from build123d import *

# Parameters (mm, degrees)
M4X0_7_TAPPED_HOLE1_D           = 3.3
M4X0_7_TAPPED_HOLE1_CSINK_D     = 8
M4X0_7_TAPPED_HOLE1_CSINK_ANGLE = 90


with BuildPart() as part:
    # Sketch2 → Revolve1 (revolve)
    with BuildSketch(Plane.XY):
        Polygon((-14, 40), (6, 40), (6, 16), (2, 16), (2, 21), (0, 21), (0, 23.5), (-4, 23.5), (-4, 35), (-14, 35), align=None)
    revolve(axis=Axis((-28.224413871, 0, 0), (1, 0, 0)))

    # M4x0.7 Tapped Hole1 (through all)
    with Locations(Plane(origin=(6, 0, 0), x_dir=(0, 0, -1), z_dir=(1, 0, 0))):
        with Locations((0, 30.5), (30.5, 0), (0, -30.5), (-30.5, 0)):
            CounterSinkHole(M4X0_7_TAPPED_HOLE1_D / 2, M4X0_7_TAPPED_HOLE1_CSINK_D / 2, counter_sink_angle=M4X0_7_TAPPED_HOLE1_CSINK_ANGLE)


solid = part.part
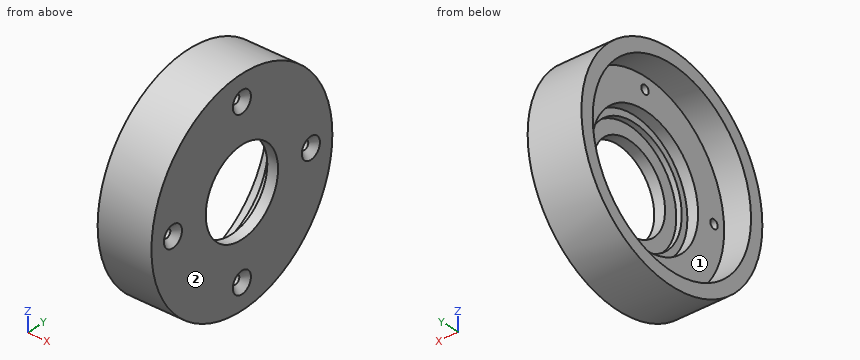
CAD build for the part. Positions are in the model's coordinates, mm. Face numbers are marked on the shaded views. A direction names the side the tool comes from. Round coordinates to 2 decimals unless told otherwise and drop trailing zeros. Loops run counter-clockwise (first coordinate to the right, second up) from the corner with the lowest first, then second, coordinate; pieces in that order, holes last. Notation, with made-up numbers: M 3,61 L 8,61 A23 cw 8,78 Z; hole C -1,11.25 d5. An arc over 180 degrees is marked long. One line per question, with ' | ' between items. Start each with the question number.
Item 1: Wall check: line 1 (Z direction, x = 3.1, y = 0); line 2 (Z direction, x = 0.5, y = 0); line 3 (Z direction, x = 1.75, y = 30.5). Give the ranges that are in metal, low to high.
Item 2: Which spindle directions (+Z, -Z, +X, -X, +Y, -Y) get a long thin tool onto all of the face, cutting with end or side? Do the marked faces 1 and 2. Say none if no direction does.
Item 3: Pin check, flat tips, straight feed: pin 1 Ø2 at (x, y) = (-8.5, 19.5) entering from +Z; pin 2 Ø2 at (x, z) = (-8.5, 21) entering from +Y; pin 3 Ø1.5 at (x, z) = (-3.5, -20) entering from +Y. Stop position of each tip, or through.
Item 4: Cut at B-B, the plane y = -30.5. Write the cut outline in (x, z).
Item 5: Cut at A-A, the plane z = 0. State how many separate pieces and enclosed holes the cut face has, plus the area to 3 significant figures.
Item 6: Cut at C-C, the plane x = -2.5. Write the cut outline in (y, z).
Responses:
1) line 1: z = -40 to -32.15, -28.85 to -16, 16 to 28.85, 32.15 to 40 | line 2: z = -40 to -32.15, -28.85 to -21, 21 to 28.85, 32.15 to 40 | line 3: z = -25.88 to -1.65, 1.65 to 25.88
2) face 1: -X | face 2: +Z, -Z, +X, +Y, -Y
3) pin 1: stops at z = 35.46 | pin 2: stops at y = 34.64 | pin 3: stops at y = 35.06
4) outline: M -14,-25.88 L 6,-25.88 L 6,-4 L 3.65,-1.65 L -4,-1.65 L -4,-17.17 L -14,-17.17 Z; M -14,17.17 L -4,17.17 L -4,1.65 L 3.65,1.65 L 6,4 L 6,25.88 L -14,25.88 Z
5) separate pieces: 4 | enclosed holes: 0 | area: 423 mm²
6) outline: C 0,0 d80; hole C -30.5,0 d3.3; hole C 0,0 d47; hole C 0,-30.5 d3.3; hole C 0,30.5 d3.3; hole C 30.5,0 d3.3
